For this review, take the finished solid that the model builds, in its own axes (mm). A direction names the side the tool comes from. Give positions to 0.01 mm unless a question says otherwise; leave off trailing zeros. Order: outer loops, then holes, each group sorted by start corner. A loop starts at its lowest first (then second) coordinate and runs counter-clockwise, first axis right, second up. Notation, with made-up numbers: M 9.25,1 L 15.25,1 A16 cw 15.25,19 Z; hole C 16,-17.5 d8. An arc over 180 degrees is marked long. Use CSV: the item, a comma, the result in double quotes. Start each with the question number.
(1) Consider section D-D (z = -7.5). Write out the cut boundary in (x, y).
(2) Consider section A-A (x = 0). Write out the cut boundary in (y, z), and give its area (3 significant figures).
(3) Draft analysis for pull direction X (two halves, no side actions). For faces 6 (the face through (-0.45, 50.42, -1.43)), 7 (the face through (2.5, 43, -0.1)), 8 (the face through (6.79, 39.3, -0.21)), state which applies: pulls with the +X half, pulls with the -X half, needs draft (parallel to the pull), parting line crosses it, or undercut.
(4) Clearance check with flat-ended pins moving along their axes: P1, Ø3, axis at y = -3, z = -0.5, coming from the +X side (3 decimals); P2, Ø5, axis at y = 11, z = 2, coming from the +X side; P3, Ø2, axis at x = 2, y = 20.5, coming from the -Z side; P4, Ø10, axis at x = 7, z = 8.5, coming from the +Y side. State where each tip first meets the part, or that it passes through.
(5) Consider section C-C (y = 8). Write out the cut boundary in (x, z), and give its area (3 significant figures).
(6) Wall thickness on L1, parallel to X at y = 37.25, z = 0; L2, parallel to Y at x = 7.8, z = 0; L3, parallel to X at y = 33, z = 0: over which ranges is each line inside the solid? List them lowest first. Write a range as from..to.
(7) Consider section B-B (y = 40.5). Write out the cut boundary in (x, z).
(8) Tool access review of faces 1 (the face through (-7.875, -4, 0)), 2 (the face through (7.625, -4, 0)), 3 (the face through (0, 56, 0)), 4 (the face through (-8, 35.5, 0)), 5 (the face through (7.875, -4, 0)): name each direction out of +Z, -Z, +X, -X, +Y, -Y from which nothing blocks a thin tool from reaching the whole face with its end or side.
```python
from build123d import *

# Parameters (mm, degrees)
SKETCH1_R           = 10.5
BOSS_EXTRUDE1_DEPTH = 43
SKETCH2_R           = 1.5
BOSS_EXTRUDE2_DEPTH = 13
SKETCH3_R           = 2.25
BOSS_EXTRUDE3_DEPTH = 2
SKETCH4_R           = 0.98394946
SKETCH4_R_2         = 1
CUT_EXTRUDE1_DEPTH  = 7.5
SKETCH5_W           = 0.25
SKETCH5_H           = 4
BOSS_EXTRUDE4_DEPTH = 1.25
SKETCH6_W           = 0.25
SKETCH6_H           = 3.55
BOSS_EXTRUDE5_DEPTH = 6
FILLET1_R           = 1
SKETCH7_R           = 0.5
CUT_EXTRUDE2_DEPTH  = 2
SKETCH8_W           = 0.25
SKETCH8_H           = 3.54
BOSS_EXTRUDE6_DEPTH = 6
FILLET2_R           = 1
SKETCH9_R           = 0.5
CUT_EXTRUDE3_DEPTH  = 3


with BuildPart() as part:
    # Sketch1 → Boss-Extrude1 (new body)
    with BuildSketch(Plane(origin=(0, 0, 0), x_dir=(1, 0, 0), z_dir=(0, 1, 0))):
        with Locations(Location((0, 0, 0), (0, 0, 270))):
            Circle(SKETCH1_R)
    extrude(amount=BOSS_EXTRUDE1_DEPTH)

    # Sketch2 → Boss-Extrude2 (add)
    with BuildSketch(Plane(origin=(0, 43, 0), x_dir=(1, 0, 0), z_dir=(0, 1, 0))):
        with Locations(Location((0, 0, 0), (0, 0, 90))):
            Circle(SKETCH2_R)
    extrude(amount=BOSS_EXTRUDE2_DEPTH)

    # Sketch3 → Boss-Extrude3 (add)
    with BuildSketch(Plane(origin=(0, 43, 0), x_dir=(1, 0, 0), z_dir=(0, 1, 0))):
        with Locations(Location((0, 0, 0), (0, 0, 270))):
            Circle(SKETCH3_R)
    extrude(amount=BOSS_EXTRUDE3_DEPTH)

    # Sketch4 → Cut-Extrude1 (cut)
    with BuildSketch(Plane(origin=(0, 43, 0), x_dir=(1, 0, 0), z_dir=(0, 1, 0))):
        with Locations(Location((7.75, 0, 0), (0, 0, 270))):
            Circle(SKETCH4_R)
        with Locations(Location((-7.75, 0, 0), (0, 0, 270))):
            Circle(SKETCH4_R_2)
    extrude(amount=-CUT_EXTRUDE1_DEPTH, mode=Mode.SUBTRACT)

    # Sketch5 → Boss-Extrude4 (add)
    with BuildSketch(Plane.XZ):
        with Locations((7.75, 0)):
            Rectangle(SKETCH5_W, SKETCH5_H)
        with Locations((-7.75, 0)):
            Rectangle(SKETCH5_W, SKETCH5_H)
    extrude(amount=BOSS_EXTRUDE4_DEPTH)

    # Sketch6 → Boss-Extrude5 (add)
    with BuildSketch(Plane.XZ.offset(1.25)):
        with Locations((-7.75, 0)):
            Rectangle(SKETCH6_W, SKETCH6_H)
    extrude(amount=BOSS_EXTRUDE5_DEPTH)

    # Fillet1
    fillet1_edges = [part.edges().sort_by_distance(p)[0] for p in [
        (-7.75, -7.25, 1.775),
        (-7.75, -7.25, -1.775),
    ]]
    fillet(fillet1_edges, radius=FILLET1_R)

    # Sketch7 → Cut-Extrude2 (cut)
    with BuildSketch(Plane.ZY.offset(7.875)):
        with Locations((0, -5.696270768)):
            Circle(SKETCH7_R)
    extrude(amount=-CUT_EXTRUDE2_DEPTH, mode=Mode.SUBTRACT)

    # Sketch8 → Boss-Extrude6 (add)
    with BuildSketch(Plane.XZ.offset(1.25)):
        with Locations((7.75, 0)):
            Rectangle(SKETCH8_W, SKETCH8_H)
    extrude(amount=BOSS_EXTRUDE6_DEPTH)

    # Fillet2
    fillet2_edges = [part.edges().sort_by_distance(p)[0] for p in [
        (7.75, -7.25, -1.77),
        (7.75, -7.25, 1.77),
    ]]
    fillet(fillet2_edges, radius=FILLET2_R)

    # Sketch9 → Cut-Extrude3 (cut)
    with BuildSketch(Plane(origin=(7.875, 0, 0), x_dir=(0, 0, -1), z_dir=(1, 0, 0))):
        with Locations((0, -5.7)):
            Circle(SKETCH9_R)
    extrude(amount=-CUT_EXTRUDE3_DEPTH, mode=Mode.SUBTRACT)


solid = part.part
```
Check result:
1,outline,"M -7.35,0 L 7.35,0 L 7.35,43 L -7.35,43 Z"
2,outline,"M 0,-10.5 L 43,-10.5 L 43,-2.25 L 45,-2.25 L 45,-1.5 L 56,-1.5 L 56,1.5 L 45,1.5 L 45,2.25 L 43,2.25 L 43,10.5 L 0,10.5 Z"
2,area,"945 mm^2"
3,face 6,"parting line crosses it"
3,face 7,"needs draft"
3,face 8,"undercut"
4,P1,"stops at x = 7.875"
4,P2,"stops at x = 10.5"
4,P3,"stops at z = -10.45"
4,P4,"stops at y = 43"
5,outline,"C 0,0 d21"
5,area,"346 mm^2"
6,L1,"x = -10.5..-8.75, -6.75..6.77, 8.73..10.5"
6,L2,"y = -7.25..-6.2, -5.2..35.5"
6,L3,"x = -10.5..10.5"
7,outline,"C 0,0 d21; hole C -7.75,0 d2; hole C 7.75,0 d1.97"
8,face 1,"+Z, -Z, -X, -Y"
8,face 2,"+Z, -Z, -Y"
8,face 3,"+Z, -Z, +X, -X, +Y"
8,face 4,"+Y"
8,face 5,"+Z, -Z, +X, -Y"
